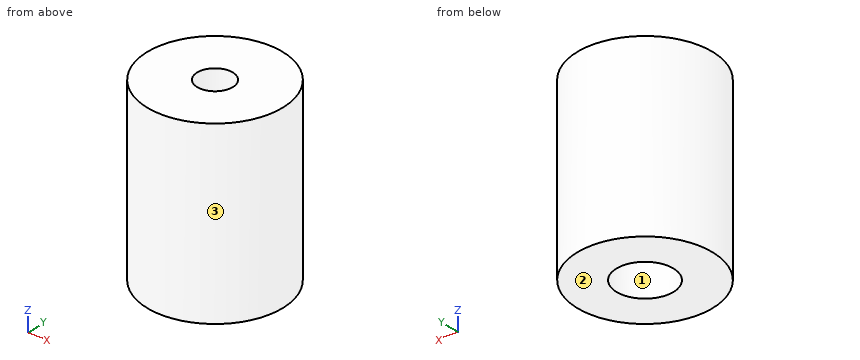
```python
from build123d import *

# Parameters (mm, degrees)
SKETCH_2_R           = 9.5
EXTRUDE_1_DEPTH      = 12.5
SKETCH_4_OUTSIDE_W   = 28.34
SKETCH_4_OUTSIDE_H   = 28.34
SKETCH_4_OUTSIDE_R   = 9.5
SKETCH_4_OUTSIDE_R_2 = 4
CUT_EXTRUDE_1_DEPTH  = 12.5
SKETCH_5_OUTSIDE_W   = 28.34
SKETCH_5_OUTSIDE_H   = 28.34
SKETCH_5_OUTSIDE_R   = 9.5
SKETCH_5_OUTSIDE_R_2 = 2.5
CUT_EXTRUDE_2_DEPTH  = 12.5


with BuildPart() as part:
    # 草图2 → 凸台-拉伸1 (new body, symmetric)
    with BuildSketch(Plane.XY.offset(10)):
        with Locations((-14.788619837, 7.492683074)):
            Circle(SKETCH_2_R)
    extrude(amount=EXTRUDE_1_DEPTH, both=True)

    # 草图4 outside → 切除-拉伸1 (cut)
    with BuildSketch(Plane.XY.offset(10)):
        with Locations((-14.789, 7.493)):
            Rectangle(SKETCH_4_OUTSIDE_W, SKETCH_4_OUTSIDE_H)
        with Locations((-14.788619837, 7.492683074)):
            Circle(SKETCH_4_OUTSIDE_R, mode=Mode.SUBTRACT)
        with Locations((-14.788619837, 7.492683074)):
            Circle(SKETCH_4_OUTSIDE_R_2)
    extrude(amount=-CUT_EXTRUDE_1_DEPTH, mode=Mode.SUBTRACT)

    # 草图5 outside → 切除-拉伸2 (cut)
    with BuildSketch(Plane.XY.offset(10)):
        with Locations((-14.789, 7.493)):
            Rectangle(SKETCH_5_OUTSIDE_W, SKETCH_5_OUTSIDE_H)
        with Locations((-14.788619837, 7.492683074)):
            Circle(SKETCH_5_OUTSIDE_R, mode=Mode.SUBTRACT)
        with Locations((-14.788619837, 7.492683074)):
            Circle(SKETCH_5_OUTSIDE_R_2)
    extrude(amount=CUT_EXTRUDE_2_DEPTH, mode=Mode.SUBTRACT)


solid = part.part
```
Part model, mm, in its own coordinate system. Face numbers are marked on the shaded views. Round coordinates to 2 decimals unless told otherwise and drop trailing zeros. Write each loop counter-clockwise with the first axis right and the second up, starting at its lowest first coordinate (ties: lowest second). Pieces come first, ordered by that corner, then holes. Notation, with made-up numbers: M 50,-31 L 60,-31 A15 cw 60,-15 Z; hole C 15,13.5 d7. An arc over 180 degrees is marked long. One line per question, with ' | ' between items.
(1) Saw through at C-C on y = 4. Write the cut outline in (x, z), then the cut area to 3 significant figures.
Answer key:
outline: M -23.62,-2.5 L -16.74,-2.5 L -16.74,10 L -12.84,10 L -12.84,-2.5 L -5.95,-2.5 L -5.95,22.5 L -23.62,22.5 Z | area: 393 mm^2
(2) Two-plate mould, pull along X, no slides. Class the marked faces 1, 2 and 3: released by +X, released by -X, zero draft, split by the parting line, or undercut.
Answer key:
face 1: undercut | face 2: zero draft | face 3: split by the parting line
(3) Saw through at A-A on y = 9.25. Write the cut outline in (x, z).
Answer key:
outline: M -24.12,-2.5 L -18.38,-2.5 L -18.38,10 L -16.57,10 L -16.57,22.5 L -24.12,22.5 Z; M -13.01,10 L -11.2,10 L -11.2,-2.5 L -5.45,-2.5 L -5.45,22.5 L -13.01,22.5 Z
(4) Saw through at B-B on x = -14.5. Write the cut outline in (y, z).
Answer key:
outline: M -2,-2.5 L 3.5,-2.5 L 3.5,10 L 5.01,10 L 5.01,22.5 L -2,22.5 Z; M 9.98,10 L 11.48,10 L 11.48,-2.5 L 16.99,-2.5 L 16.99,22.5 L 9.98,22.5 Z
(5) Saw through at D-D on z = 13.75. Write the cut outline in (x, y), then the cut area to 3 significant figures.
Answer key:
outline: C -14.79,7.49 d19; hole C -14.79,7.49 d5 | area: 264 mm^2
(6) Pin check, flat tips, straight feed: pin 1 (5 mm diameter, centred on y = 0.5, z = 18.5, fed in from -X); pin 2 (8 mm diameter, centred on x = -9, z = 18.5, fed in from -Y); pin 3 (4 mm diameter, centred on y = 0.5, z = 3.5, fed in from +X); pin 4 (4 mm diameter, centred on x = -14.79, y = 7.49, fed in from +Z). Stop position of each tip, or through.
Answer key:
pin 1: stops at x = -23.16 | pin 2: stops at y = -1.84 | pin 3: stops at x = -6.71 | pin 4: passes through
(7) Probe line 1 along Y through (x, z) = (-16.5, -0.5); line 2 along X through (y, z) = (6, 1); line 3 along Y through (x, z) = (-16, 14.5). List the from-to ranges inside material, lowest first.
Answer key:
line 1: y = -1.85 to 3.88, 11.11 to 16.84 | line 2: x = -24.17 to -18.5, -11.08 to -5.41 | line 3: y = -1.93 to 5.31, 9.68 to 16.92
